Build history of the part. All positions in model axes, mm. Face numbers are marked on the shaded views. Give positions to 0.01 mm unless a question says otherwise; leave off trailing zeros. Write each loop counter-clockwise with the first axis right and the second up, starting at its lowest first coordinate (ties: lowest second). Pieces come first, ordered by that corner, then holes.
from build123d import *

# Parameters (mm, degrees)
F0_R     = 9.95
F1_DEPTH = 6


with BuildPart() as f1:
    # F0 (on Top) → F1 (new body)
    with BuildSketch(Plane.XY):
        with BuildLine():
            ThreePointArc((21.557813, 2.499713), (14.522567, 7.888802), (12.344861, 16.479178))
            ThreePointArc((12.344861, 16.479178), (0.911041, 39.972308), (-13.286915, 18.03883))
            ThreePointArc((-13.286915, 18.03883), (-13.935579, 9.012352), (-20.139405, 2.423679))
            ThreePointArc((-20.139405, 2.423679), (-34.833486, -19.656287), (-8.312649, -19.362807))
            ThreePointArc((-8.312649, -19.362807), (0, -16.5), (8.312649, -19.362807))
            ThreePointArc((8.312649, -19.362807), (34.479863, -20.272445), (21.557813, 2.499713))
        make_face()
        with Locations((-21.650635, -12.5)):
            Circle(F0_R, mode=Mode.SUBTRACT)
        with Locations((21.650635, -12.5)):
            Circle(F0_R, mode=Mode.SUBTRACT)
        with BuildLine():
            ThreePointArc((0, 11), (7.778175, 7.778175), (11, 0))
            ThreePointArc((11, 0), (7.778175, -7.778175), (0, -11))
            ThreePointArc((0, -11), (-11, 0), (0, 11))
        make_face(mode=Mode.SUBTRACT)
        with Locations((0, 25)):
            Circle(F0_R, mode=Mode.SUBTRACT)
    extrude(amount=F1_DEPTH)


solid = f1.part
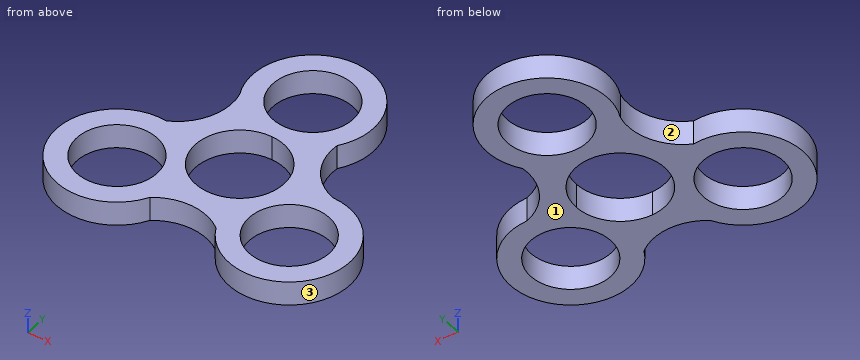
1. Mould opens along Y. For the marked faces 1, 2 and 3 say: pulls with the +Y half, pulls with the -Y half, needs draft (parallel to the pull), parting line crosses it, or undercut.
2. Saw through at A-A on y = -12.5. Give the cut face in (x, z).
3. Saw through at D-D on x = 4.5. Give the cut face in (y, z).
4. Saw through at B-B on y = 25. Give the cut face in (x, z).
5. Drop flat-ended pins along their axis: pin 1 (12 mm diameter, centred on x = -22, y = 21.5, fed in from +Z); pin 2 (3 mm diameter, centred on y = 22, z = 4.5, fed in from -X); pin 3 (1.5 mm diameter, centred on y = 1, z = 1, fed in from -X). Give the stop position or say it passes through.
6. Drill centre lines: line 1 along X through (y, z) = (-12, 2.05); line 2 along Y through (x, z) = (-2, 2.95); line 3 along X through (y, z) = (-14, 0.95). Where is each one in solid material? Low to high.
7. Saw through at C-C on x = 28. Give the cut face in (y, z).
Outcome:
1. face 1: needs draft
1. face 2: undercut
1. face 3: parting line crosses it
2. outline: (-36.65, 0) - (-31.6, 0) - (-31.6, 6) - (-36.65, 6) - close; (-11.7, 0) - (11.7, 0) - (11.7, 6) - (-11.7, 6) - close; (31.6, 0) - (36.65, 0) - (36.65, 6) - (31.6, 6) - close
3. outline: (-17.27, 0) - (-10.04, 0) - (-10.04, 6) - (-17.27, 6) - close; (10.04, 0) - (16.13, 0) - (16.13, 6) - (10.04, 6) - close; (33.87, 0) - (39.31, 0) - (39.31, 6) - (33.87, 6) - close
4. outline: (-15, 0) - (-9.95, 0) - (-9.95, 6) - (-15, 6) - close; (9.95, 0) - (15, 0) - (15, 6) - (9.95, 6) - close
5. pin 1: passes through
5. pin 2: stops at x = -14.92
5. pin 3: stops at x = -29.55
6. line 1: x = -36.64 to -31.59, -11.71 to 11.71, 31.59 to 36.64
6. line 2: y = -16.65 to -10.82, 10.82 to 15.25, 34.75 to 39.87
6. line 3: x = -36.58 to -31.49, -11.81 to 11.81, 31.49 to 36.58
7. outline: (-26.09, 0) - (-20.16, 0) - (-20.16, 6) - (-26.09, 6) - close; (-4.84, 0) - (1.09, 0) - (1.09, 6) - (-4.84, 6) - close
